from build123d import *

# Parameters (mm, degrees)
SKETCH1_W           = 39
SKETCH1_H           = 45
BOSS_EXTRUDE1_DEPTH = 12.5
SKETCH2_R           = 4.05
CUT_EXTRUDE1_DEPTH  = 61.846117378
SKETCH3_W           = 50
SKETCH3_H           = 50
BOSS_EXTRUDE2_DEPTH = 5.5
BOSS_EXTRUDE3_START = -10
BOSS_EXTRUDE3_DEPTH = 5
LPATTERN1_COUNT     = 2
LPATTERN1_PITCH     = 14
FILLET1_R           = 5
SKETCH5_R           = 1.6
CUT_EXTRUDE2_DEPTH  = 79.17008699
FILLET2_R           = 20
CUT_EXTRUDE3_DEPTH  = 73.615855707
CUT_EXTRUDE4_START  = -1
SKETCH7_W           = 39.2
SKETCH7_H           = 50.063664736
SKETCH7_R           = 11
SKETCH7_W_2         = 11
SKETCH7_H_2         = 11
CUT_EXTRUDE4_DEPTH  = 1
SKETCH8_W           = 25
SKETCH8_H           = 5
SKETCH8_W_2         = 5
SKETCH8_H_2         = 25
BOSS_EXTRUDE4_DEPTH = 0.5


with BuildPart() as part:
    # Sketch1 → Boss-Extrude1 (new body)
    with BuildSketch(Plane(origin=(0, 0, 0), x_dir=(1, 0, 0), z_dir=(0, 1, 0))):
        with Locations((19.5, 22.5)):
            Rectangle(SKETCH1_W, SKETCH1_H)
    extrude(amount=BOSS_EXTRUDE1_DEPTH)

    # Sketch2 → Cut-Extrude1 (cut, through all)
    with BuildSketch(Plane(origin=(0, 12.5, 0), x_dir=(1, 0, 0), z_dir=(0, 1, 0))):
        with Locations(Location((19.5, 15, 0), (0, 0, 270))):
            Circle(SKETCH2_R)
    extrude(amount=-CUT_EXTRUDE1_DEPTH, mode=Mode.SUBTRACT)

    # Sketch3 → Boss-Extrude2 (add)
    with BuildSketch(Plane(origin=(0, 0, -45), x_dir=(-1, 0, 0), z_dir=(0, 0, -1))):
        with Locations((-19.5, 14.75)):
            Rectangle(SKETCH3_W, SKETCH3_H)
    extrude(amount=BOSS_EXTRUDE2_DEPTH)

    # Sketch4 → Boss-Extrude3 (add)
    with BuildSketch(Plane(origin=(39, 0, 0), x_dir=(0, 0, -1), z_dir=(1, 0, 0)).offset(BOSS_EXTRUDE3_START)):
        Polygon((33, 12.5), (45, 24.5), (45, 12.5), align=None)
    boss_extrude3 = extrude(amount=-BOSS_EXTRUDE3_DEPTH)

    # LPattern1: Boss-Extrude3 ×2
    with Locations(*[(-i * LPATTERN1_PITCH, 0, 0) for i in range(1, LPATTERN1_COUNT)]):
        add(boss_extrude3)

    # Fillet1
    fillet1_edges = [part.edges().sort_by_distance(p)[0] for p in [
        (26.5, 12.5, -33),
        (26.5, 24.5, -45),
        (12.5, 12.5, -33),
        (12.5, 24.5, -45),
    ]]
    fillet(fillet1_edges, radius=FILLET1_R)

    # Sketch5 → Cut-Extrude2 (cut, through all)
    with BuildSketch(Plane(origin=(0, 0, -50.5), x_dir=(-1, 0, 0), z_dir=(0, 0, -1))):
        with Locations((-37.5, 32.75)):
            Circle(SKETCH5_R)
        with Locations((-1.5, 32.75)):
            Circle(SKETCH5_R)
        with Locations((-1.5, -3.25)):
            Circle(SKETCH5_R)
        with Locations((-37.5, -3.25)):
            Circle(SKETCH5_R)
    extrude(amount=-CUT_EXTRUDE2_DEPTH, mode=Mode.SUBTRACT)

    # Fillet2
    # the kernel refuses this fillet: 20 mm, written as the material it takes off along each edge
    with BuildSketch(Plane(origin=(0, -50, 0), x_dir=(0, 0, -1), z_dir=(0, 1, 0))) as fillet2_piece_1:
        with BuildLine():
            CenterArc((FILLET2_R, -FILLET2_R), FILLET2_R, 90, 90)
            Line((0, -FILLET2_R), (0, 0))
            Line((0, 0), (FILLET2_R, 0))
        make_face()
    extrude(amount=112.5, mode=Mode.SUBTRACT)
    with BuildSketch(Plane(origin=(39, -50, 0), x_dir=(0, 0, -1), z_dir=(0, 1, 0))) as fillet2_piece_2:
        with BuildLine():
            CenterArc((FILLET2_R, FILLET2_R), FILLET2_R, 180, 90)
            Line((0, FILLET2_R), (0, 0))
            Line((0, 0), (FILLET2_R, 0))
        make_face()
    extrude(amount=112.5, mode=Mode.SUBTRACT)

    # Sketch6 → Cut-Extrude3 (cut, through all)
    with BuildSketch(Plane(origin=(0, 12.5, 0), x_dir=(1, 0, 0), z_dir=(0, 1, 0))):
        with BuildLine():
            Line((7, 20), (7, 28.347560338))
            Line((7, 28.347560338), (15.5, 28.347560338))
            Line((15.5, 28.347560338), (15.5, 25.246950766))
            ThreePointArc((15.5, 25.246950766), (10.417048938, 21.204836823), (8.5, 15))
            ThreePointArc((8.5, 15), (7.383077909, 17.389923373), (7, 20))
        make_face()
        with BuildLine():
            Line((23.5, 25.246950766), (23.5, 28.347560338))
            Line((23.5, 28.347560338), (32, 28.347560338))
            Line((32, 28.347560338), (32, 20))
            ThreePointArc((32, 20), (31.605614865, 17.768951725), (30.47026085, 15.808317311))
            ThreePointArc((30.47026085, 15.808317311), (28.348679441, 21.534590434), (23.5, 25.246950766))
        make_face()
    extrude(amount=-CUT_EXTRUDE3_DEPTH, mode=Mode.SUBTRACT)

    # Sketch7 → Cut-Extrude4 (cut)
    with BuildSketch(Plane.XZ.offset(CUT_EXTRUDE4_START)):
        with Locations((19.5, -19.968167632)):
            Rectangle(SKETCH7_W, SKETCH7_H)
        with Locations(Location((19.5, -15, 0), (0, 0, 180))):
            Circle(SKETCH7_R, mode=Mode.SUBTRACT)
        with Locations((10, -37.501795484)):
            Rectangle(SKETCH7_W_2, SKETCH7_H_2, mode=Mode.SUBTRACT)
        with Locations((29, -37.501795484)):
            Rectangle(SKETCH7_W_2, SKETCH7_H_2, mode=Mode.SUBTRACT)
    extrude(amount=CUT_EXTRUDE4_DEPTH, mode=Mode.SUBTRACT)

    # Sketch8 → Boss-Extrude4 (add)
    with BuildSketch(Plane(origin=(0, 0, -50.5), x_dir=(-1, 0, 0), z_dir=(0, 0, -1))):
        with Locations((-19.5, 32.75)):
            Rectangle(SKETCH8_W, SKETCH8_H)
        with Locations((-1.5, 14.75)):
            Rectangle(SKETCH8_W_2, SKETCH8_H_2)
        with Locations((-19.5, -3.25)):
            Rectangle(SKETCH8_W, SKETCH8_H)
        with Locations((-37.5, 14.75)):
            Rectangle(SKETCH8_W_2, SKETCH8_H_2)
    extrude(amount=BOSS_EXTRUDE4_DEPTH)


solid = part.part
Design review of the part built by this model. Coordinates are the model's own, in mm. A direction names the side the tool comes from. Give positions to 0.01 mm unless a question says otherwise; leave off trailing zeros. Loops run counter-clockwise (first coordinate to the right, second up) from the corner with the lowest first, then second, coordinate; pieces in that order, holes last. Notation, with made-up numbers: (-28.75, -5) - (6.25, -5) arc R28 ccw to (6.25, 34) - close; hole circle Ø3 at (-11, 40). An arc over 180 degrees is marked (long way). Write item = value, one per line.
1) Draft analysis for pull direction Y (two halves, no side actions). For faces 6 (the face through (38, 15, -51)), 7 (the face through (1.85, 31.19, -47.79)), 8 (the face through (24, 0, -15)), state which applies: +Y half, -Y half, draft (parallel to the pull), parting line (faces both ways), or undercut.
Result sheet:
face_6 = draft
face_7 = undercut
face_8 = -Y half
2) To check wall thickness, follow line 1 (Y direction, x = 37.5, z = -48.2); line 2 (Y direction, x = 28, z = -12.5); line 3 (Z direction, x = 7.5, y = 37.5). State the ranges of each line that lie inside material, in increasing order.
Result sheet:
line_1 = -10.25 to -4.85, -1.65 to 31.15, 34.35 to 39.75
line_2 = 0 to 12.5
line_3 = -50.5 to -45
3) Tool access review of faces 1 (the face through (10, 0, -38)), 2 (the face through (23.5, 7, -27)), 3 (the face through (15, 16, -41)), 4 (the face through (20, -10.25, -48)), 5 (the face through (29, 16, -41)): name each direction out of +Z, -Z, +X, -X, +Y, -Y from which nothing blocks a thin tool from reaching the whole face with its end or side.
Result sheet:
face_1 = +Z, +X, -X, -Y
face_2 = +Y, -Y
face_3 = +Z, +Y
face_4 = +Z, -Z, +X, -X, -Y
face_5 = +Z, +X, +Y
4) Take a section at B-B on z = -12. State the section outline as (x, y) points.
Result sheet:
outline = (1.67, 1) - (8.92, 1) - (8.92, 0) - (16.78, 0) - (16.78, 12.5) - (1.67, 12.5) - close; (22.22, 0) - (30.08, 0) - (30.08, 1) - (37.33, 1) - (37.33, 12.5) - (22.22, 12.5) - close
5) Take a section at C-C on x = 22. State the section outline as (y, z) points.
Result sheet:
outline = (-10.25, -50.5) - (-5.75, -50.5) - (-5.75, -51) - (-0.75, -51) - (-0.75, -50.5) - (30.25, -50.5) - (30.25, -51) - (35.25, -51) - (35.25, -50.5) - (39.75, -50.5) - (39.75, -45) - (12.5, -45) - (12.5, -18.19) - (0, -18.19) - (0, -25.71) - (1, -25.71) - (1, -45) - (-10.25, -45) - close; (0, -11.81) - (12.5, -11.81) - (12.5, -0.23) - (1, -0.23) - (1, -4.29) - (0, -4.29) - close
6) Take a section at D-D on z = -38.5. State the section outline as (x, y) points, and give its area (4 significant figures).
Result sheet:
outline = (0, 1) - (4.5, 1) - (4.5, 0) - (15.5, 0) - (15.5, 1) - (23.5, 1) - (23.5, 0) - (34.5, 0) - (34.5, 1) - (39, 1) - (39, 12.5) - (29, 12.5) - (29, 18) - (24, 18) - (24, 12.5) - (15, 12.5) - (15, 18) - (10, 18) - (10, 12.5) - (0, 12.5) - close
area = 525.5 mm2
7) Take a section at A-A on y = -3.25. State the section outline as (x, z) points, and give its area (3 significant figures).
Result sheet:
outline = (-5.5, -50.5) - (-0.1, -50.5) - (-0.1, -45) - (-5.5, -45) - close; (3.1, -50.5) - (7, -50.5) - (7, -51) - (32, -51) - (32, -50.5) - (35.9, -50.5) - (35.9, -45) - (3.1, -45) - close; (39.1, -50.5) - (44.5, -50.5) - (44.5, -45) - (39.1, -45) - close
area = 252 mm2
8) Clearance check with flat-ended pins moving along their axes: pin 1 Ø4 at (x, y) = (21.5, 16) entering from -Z; pin 2 Ø5 at (x, z) = (10, -34.5) entering from -Y; pin 3 Ø1.5 at (y, z) = (12, -10.5) entering from +X. State where each tip first meets the part, or that it passes through.
Result sheet:
pin_1 = -50.5
pin_2 = 0
pin_3 = 36.98
